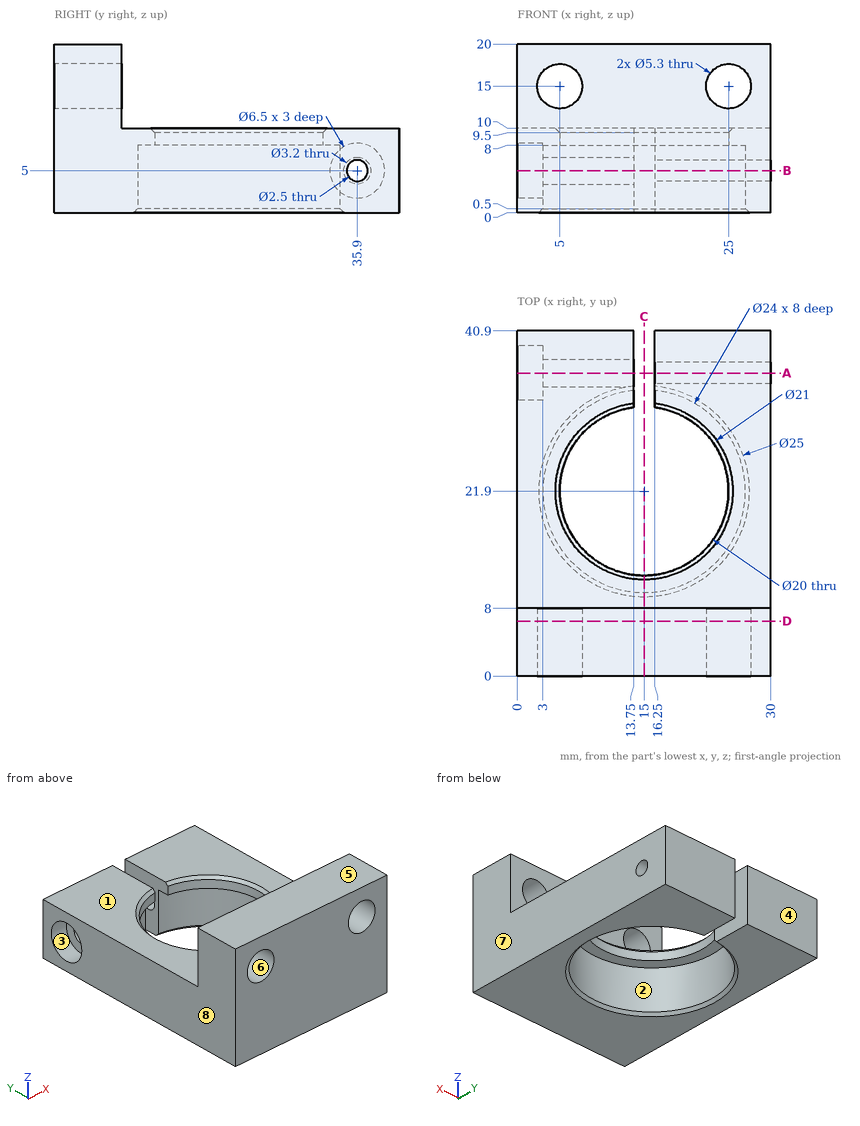
Answer from the drawing. Dimensions are ordinates in mm from the lowest x, y and z of the part. A direction names the side the tool comes from. Round coordinates to 2 decimals unless told otherwise and drop trailing zeros. Order: outer loops, then holes, each group sorted by start corner. A loop starts at its lowest first (then second) coordinate and runs counter-clockwise, first axis right, second up. Notation, with made-up numbers: (-2.5, -23) - (2.5, -23) arc R30 ccw to (2.5, -1) - close; hole circle Ø11 at (-39.75, -23.5). An arc over 180 degrees is marked (long way). Put each result on its own line as item: value. Start each with the question number.
(1) For the marked faces 1, 2, 3 and 4, determine the directions among +Z, -Z, +X, -X, +Y, -Y from which every point of the face is accessible in a straight line to the end or side of a thin tool.
(2) Find section D-D (y = 6.5). Give the vertices of the cut face in (x, z).
(3) Find section B-B (z = 5). Give the vertices of the cut face in (x, y), plus the area to 3 significant figures.
(4) Determine the mould class of the marked faces 5, 6, 7 and 8 for opening direction X: released by +X, released by -X, zero draft, split by the parting line, or undercut.
(5) Given P1, Ø3, axis at y = 35.9, z = 5, coming from the -X side; P2, Ø5, axis at y = 35.9, z = 5, coming from the -X side; P3, Ø5, axis at x = 18, z = 17.5, coming from the +Y side, each flat-ended and moving along its own axis, determine where each tip first touches the part or whether it passes through.
(6) Straight lines are drawn through the part: probe 1 along X at (y, z) = (5, 15); probe 2 along Z at (x, y) = (5, 2.75); probe 3 along X at (y, z) = (22, 5.5). For each, find the intervals that lie inside material, in ascending order. Write a range as from..to.
(7) Find section A-A (y = 35.9). Give the vertices of the cut face in (x, z), plus the area to 3 significant figures.
(8) Find section C-C (x = 15). Give the vertices of the cut face in (y, z).
Reply:
1. face 1: +Z, +X, -X, +Y
1. face 2: -Z
1. face 3: -X
1. face 4: +Z, -Z, +X, -X, +Y
2. outline: (0, 0) - (30, 0) - (30, 20) - (0, 20) - close; hole circle Ø5.3 at (5, 15); hole circle Ø5.3 at (25, 15)
3. outline: (0, 0) - (30, 0) - (30, 34.65) - (16.25, 34.65) - (16.25, 33.83) arc R12 cw (long way) to (13.75, 33.83) - (13.75, 34.3) - (3, 34.3) - (3, 32.65) - (0, 32.65) - close; (0, 39.15) - (3, 39.15) - (3, 37.5) - (13.75, 37.5) - (13.75, 40.9) - (0, 40.9) - close; (16.25, 37.15) - (30, 37.15) - (30, 40.9) - (16.25, 40.9) - close
3. area: 669 mm^2
4. face 5: zero draft
4. face 6: undercut
4. face 7: released by +X
4. face 8: released by -X
5. P1: x = 16.25
5. P2: x = 3
5. P3: y = 8
6. probe 1: 0..2.35, 7.65..22.35, 27.65..30
6. probe 2: 0..12.35, 17.65..20
6. probe 3: 0..3, 27..30
7. outline: (0, 0) - (13.75, 0) - (13.75, 3.4) - (3, 3.4) - (3, 1.75) - (0, 1.75) - close; (0, 8.25) - (3, 8.25) - (3, 6.6) - (13.75, 6.6) - (13.75, 10) - (0, 10) - close; (16.25, 0) - (30, 0) - (30, 3.75) - (16.25, 3.75) - close; (16.25, 6.25) - (30, 6.25) - (30, 10) - (16.25, 10) - close
7. area: 187 mm^2
8. outline: (0, 0) - (9.4, 0) - (9.9, 0.5) - (9.9, 8) - (11.9, 8) - (11.9, 9.5) - (11.4, 10) - (8, 10) - (8, 20) - (0, 20) - close
